Source: CAD feature listing. Evaluate the final solid. Frame: model axes, mm. A direction names the side the tool comes from. Give positions to 0.01 mm unless a question says otherwise; leave off trailing zeros. Loops run counter-clockwise (first coordinate to the right, second up) from the corner with the lowest first, then second, coordinate; pieces in that order, holes last. Notation, with made-up numbers: (-33, 64) - (23, 64) arc R22 ccw to (23, 101) - close; hole circle Ø7 at (64, -27). An arc over 180 degrees is marked (long way). Put each result on its own line as item: value.
```python
from build123d import *

# Parameters (mm, degrees)
BOSS_EXTRUDE1_DEPTH = 5
SKETCH2_W           = 1.1
SKETCH2_H           = 4.6
BOSS_EXTRUDE2_DEPTH = 3
CUT_EXTRUDE1_REACH  = 9.993


with BuildPart() as part:
    # Sketch1 → Boss-Extrude1 (new body)
    with BuildSketch(Plane(origin=(0, 0, 0), x_dir=(1, 0, 0), z_dir=(0, 1, 0))):
        Polygon((2.25, 1.5), (0.75, 3), (-0.75, 3), (-0.75, -3), (0.75, -3), (0.75, 1.5), align=None)
    extrude(amount=BOSS_EXTRUDE1_DEPTH)

    # Sketch2 → Boss-Extrude2 (add)
    with BuildSketch(Plane.XY.offset(3)):
        with Locations((0, 2.5)):
            Rectangle(SKETCH2_W, SKETCH2_H)
    extrude(amount=BOSS_EXTRUDE2_DEPTH)

    # Sketch3 → Cut-Extrude1 (cut, up to next)
    with BuildSketch(Plane(origin=(0.55, 0, 0), x_dir=(0, 0, -1), z_dir=(1, 0, 0)), mode=Mode.PRIVATE) as cut_extrude1_sk1:
        Polygon((-6, 3.3), (-4.5, 4.8), (-6, 4.8), align=None)
    cut_extrude1_tool1 = extrude(cut_extrude1_sk1.sketch, amount=-CUT_EXTRUDE1_REACH, mode=Mode.PRIVATE) & part.part
    cut_extrude1 = cut_extrude1_tool1.solids().sort_by_distance((0.55, 4.3, 5.5))[0]
    add(cut_extrude1, mode=Mode.SUBTRACT)

    # Mirror1: Cut-Extrude1 across plane
    add(cut_extrude1.mirror(Plane.ZX.offset(2.5)), mode=Mode.SUBTRACT)


solid = part.part
```
1) Material intervals for line 1 along X through (y, z) = (1.95, 1.75); line 2 along Y through (x, z) = (0.1, 3.5); line 3 along Z through (x, y) = (-0.05, 0.5), sorted ascending. Write a range as [from, to].
Check result:
line 1: [-0.75, 0.75]
line 2: [0.2, 4.8]
line 3: [-3, 4.8]
2) Section query C-C, the plane z = 4. Output: boundary loops of the cut face in (x, y).
Check result:
outline: (-0.55, 0.2) - (0.55, 0.2) - (0.55, 4.8) - (-0.55, 4.8) - close
3) Section query A-A, the plane y = 4.7. Output: boundary loops of the cut face in (x, z), plus the area to 3 significant figures.
Check result:
outline: (-0.75, -3) - (0.75, -3) - (2.25, -1.5) - (0.75, -1.5) - (0.75, 3) - (0.55, 3) - (0.55, 4.6) - (-0.55, 4.6) - (-0.55, 3) - (-0.75, 3) - close
area: 11.9 mm²
4) Section query D-D, the plane x = 1.9. Output: boundary loops of the cut face in (y, z).
Check result:
outline: (0, -1.85) - (5, -1.85) - (5, -1.5) - (0, -1.5) - close
5) Section query B-B, the plane x = 0.45. Output: boundary loops of the cut face in (y, z).
Check result:
outline: (0, -3) - (5, -3) - (5, 3) - (4.8, 3) - (4.8, 4.5) - (3.3, 6) - (1.7, 6) - (0.2, 4.5) - (0.2, 3) - (0, 3) - close
6) Pin query (flat end, axial travel): P1, Ø1.5, axis at y = 1.5, z = 4, coming from the +X side; P2, Ø0.9, axis at x = 0, z = 3.5, coming from the +Y side; P3, Ø2.5, axis at y = 2, z = 5, coming from the -X side. Return the tip coordinate at first contact, or that it passes through.
Check result:
P1: x = 0.55
P2: y = 4.8
P3: x = -0.55
7) Access query for faces 1 (the flat face through (1.51, 2.46, -2.24)), 2 (the flat face through (0, 0.2, 4)), 3 (the flat face through (0, 4.8, 4)), 4 (the flat face through (-0.55, 2, 4)), 5 (the flat face through (1, 2, -1.5)). Directions: +Z, -Z, +X, -X, +Y, -Y. A direction counts if a zero-diameter tool reaches every point of the face in a straight line with its end or side. Return the directions, or none.
Check result:
face 1: -Z, +X, +Y, -Y
face 2: +Z, +X, -X, -Y
face 3: +Z, +X, -X, +Y
face 4: +Z, -X, +Y, -Y
face 5: +Z, +X, +Y, -Y
